from build123d import *

# Parameters (mm, degrees)
SKETCH_1_W          = 20
SKETCH_1_H          = 20
SKETCH_1_R          = 1.35
EXTRUDE_1_DEPTH     = 10
SKETCH_3_R          = 1.35
CUT_EXTRUDE_1_DEPTH = 25.494897428
FILLET_1_R          = 2


with BuildPart() as part:
    # 草图1 → 凸台-拉伸1 (new body)
    with BuildSketch(Plane(origin=(0, 0, 0), x_dir=(1, 0, 0), z_dir=(0, 1, 0))):
        Rectangle(SKETCH_1_W, SKETCH_1_H)
        with Locations(Location((0, 6, 0), (0, 0, 270))):
            Circle(SKETCH_1_R, mode=Mode.SUBTRACT)
        with Locations(Location((0, -6, 0), (0, 0, 90))):
            Circle(SKETCH_1_R, mode=Mode.SUBTRACT)
    extrude(amount=EXTRUDE_1_DEPTH)

    # 草图3 → 切除-拉伸1 (cut, through all)
    with BuildSketch(Plane(origin=(0, 0, -10), x_dir=(-1, 0, 0), z_dir=(0, 0, -1))):
        with Locations((5, 5)):
            Circle(SKETCH_3_R)
        with Locations(Location((-5, 5, 0), (0, 0, 180))):
            Circle(SKETCH_3_R)
    extrude(amount=-CUT_EXTRUDE_1_DEPTH, mode=Mode.SUBTRACT)

    # 圆角1
    fillet_1_edges = [part.edges().sort_by_distance(p)[0] for p in [
        (10, 5, 10),
        (-10, 5, 10),
        (-10, 5, -10),
        (10, 5, -10),
    ]]
    fillet(fillet_1_edges, radius=FILLET_1_R)


solid = part.part
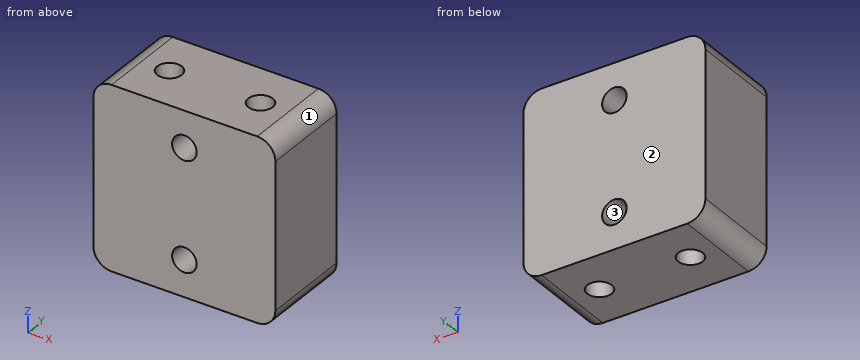
Here's how the part is built. I have some questions about the finished solid (model axes, mm). Face numbers are marked on the shaded views. Give positions to 0.01 mm unless a question says otherwise; leave off trailing zeros. Order: outer loops, then holes, each group sorted by start corner. A loop starts at its lowest first (then second) coordinate and runs counter-clockwise, first axis right, second up. Notation, with made-up numbers: (-14.75, 21) -> (21.25, 21) arc R22 ccw to (21.25, 49) -> close; hole circle Ø10 at (76.5, 42). An arc over 180 degrees is marked (long way). One line per item, written item: value. Start each with the question number.
1. I need wall thicknesses on probe 1 along Y at (x, z) = (5, 5); probe 2 along Z at (x, y) = (-0.75, 9.25); probe 3 along X at (y, z) = (5.75, 3). Which ranges of each line are inside material? Lowest first, please. Write a range as from..to.
2. Imagine slicing it at B-B, the plane z = -6. List the corners of the cut face in (x, y) for me, plus the area to 3 significant figures.
3. Imagine slicing it at A-A, the plane y = 5. List the corners of the cut face in (x, z) for me.
4. Imagine slicing it at D-D, the plane y = 1.5. List the corners of the cut face in (x, z) for me.
5. Imagine slicing it at C-C, the plane x = 0. List the corners of the cut face in (y, z) for me.
6. We'd pull the mould along X, two halves only. Please class the marked faces 1, 2 and 3: released by +X, released by -X, zero draft, split by the parting line, or undercut.
Values follow:
1. probe 1: y = 0..3.65, 6.35..10
1. probe 2: z = -10..-7.12, -4.88..4.88, 7.12..10
1. probe 3: x = -10..-6.12, -3.88..3.88, 6.12..10
2. outline: (-10, 0) -> (-1.35, 0) -> (-1.35, 10) -> (-10, 10) -> close; (1.35, 0) -> (10, 0) -> (10, 10) -> (1.35, 10) -> close; hole circle Ø2.7 at (-5, 5); hole circle Ø2.7 at (5, 5)
2. area: 162 mm2
3. outline: (-10, -8) arc R2 ccw to (-8, -10) -> (-6.35, -10) -> (-6.35, 10) -> (-8, 10) arc R2 ccw to (-10, 8) -> close; (-3.65, -10) -> (3.65, -10) -> (3.65, 10) -> (-3.65, 10) -> close; (6.35, -10) -> (8, -10) arc R2 ccw to (10, -8) -> (10, 8) arc R2 ccw to (8, 10) -> (6.35, 10) -> close; hole circle Ø2.7 at (0, -6); hole circle Ø2.7 at (0, 6)
4. outline: (-10, -8) arc R2 ccw to (-8, -10) -> (8, -10) arc R2 ccw to (10, -8) -> (10, 8) arc R2 ccw to (8, 10) -> (-8, 10) arc R2 ccw to (-10, 8) -> close; hole circle Ø2.7 at (0, -6); hole circle Ø2.7 at (0, 6)
5. outline: (0, -10) -> (10, -10) -> (10, -7.35) -> (0, -7.35) -> close; (0, -4.65) -> (10, -4.65) -> (10, 4.65) -> (0, 4.65) -> close; (0, 7.35) -> (10, 7.35) -> (10, 10) -> (0, 10) -> close
6. face 1: released by +X
6. face 2: zero draft
6. face 3: undercut
